Job drawing, mm, ordinate dimensions from the low corner. One solid piece. A direction names the side the tool comes from. Give positions to 0.01 mm unless a question says otherwise; leave off trailing zeros. Write each loop counter-clockwise with the first axis right and the second up, starting at its lowest first coordinate (ties: lowest second). Pieces come first, ordered by that corner, then holes. Notation, with made-up numbers: (40, 61) -> (70, 61) arc R21 cw to (70, 84) -> close; hole circle Ø11 at (-26.75, 18.25). An arc over 180 degrees is marked (long way). Put each result on its own line as item: value. Start each with the question number.
Item 1: Slice it at A-A, the plane x = 9.75. List the corners of the cut face in (y, z).
Item 2: Tool access for the marked faces 4 and 5: list every direction of +Z, -Z, +X, -X, +Y, -Y with a clear straight run to the whole face (end or side of a thin tool).
Item 3: Two-plate mould, pull along Y, no slides. Class the marked faces 1, 2 and 3: pulls with the +Y half, pulls with the -Y half, needs draft (parallel to the pull), parting line crosses it, or undercut.
Item 4: Slice it at D-D, the plane y = 12.25. List the corners of the cut face in (x, z).
Item 5: Slice it at C-C, the plane z = 1.15. List the corners of the cut face in (x, y).
Item 6: Flat gauge pins, fed straight in: pin 1 Ø1 at (x, z) = (9.5, 1) entering from +Y; pin 2 Ø0.8 at (y, z) = (1.5, 1) entering from -X; pin 3 Ø1.6 at (x, z) = (8, 1) entering from -Y. Where does each tip first touch, or does it go through?
Item 7: Slice it at B-B, the plane y = 1.5. List the corners of the cut face in (x, z), plus the area to 3 significant figures.
Item 8: Drill centre lines: line 1 along Y through (x, z) = (8.25, 0.3); line 2 along Z through (x, y) = (7.25, 7.5); line 3 along X through (y, z) = (5.25, 1.05). Where is each one in solid material? Low to high.
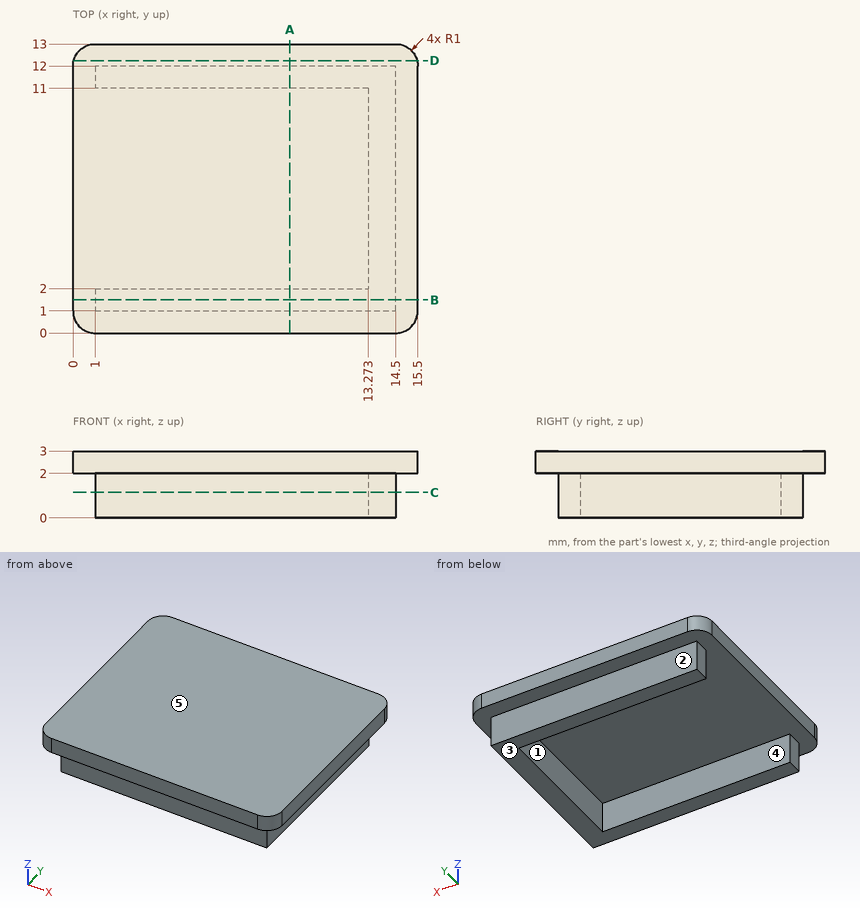
Values follow:
1. outline: (0, 2) -> (1, 2) -> (1, 0) -> (2, 0) -> (2, 2) -> (11, 2) -> (11, 0) -> (12, 0) -> (12, 2) -> (13, 2) -> (13, 3) -> (0, 3) -> close
2. face 4: -Z, -X
2. face 5: +Z, +X, -X, +Y, -Y
3. face 1: undercut
3. face 2: pulls with the +Y half
3. face 3: needs draft
4. outline: (0.03, 2) -> (15.47, 2) -> (15.47, 3) -> (0.03, 3) -> close
5. outline: (1, 1) -> (14.5, 1) -> (14.5, 12) -> (1, 12) -> (1, 11) -> (13.27, 11) -> (13.27, 2) -> (1, 2) -> close
6. pin 1: y = 12
6. pin 2: x = 1
6. pin 3: y = 1
7. outline: (0, 2) -> (1, 2) -> (1, 0) -> (14.5, 0) -> (14.5, 2) -> (15.5, 2) -> (15.5, 3) -> (0, 3) -> close
7. area: 42.5 mm2
8. line 1: 1 to 2, 11 to 12
8. line 2: 2 to 3
8. line 3: 13.27 to 14.5
